Source: CAD feature listing. Evaluate the final solid. Frame: model axes, mm. A direction names the side the tool comes from. Give positions to 0.01 mm unless a question says otherwise; leave off trailing zeros. Write each loop counter-clockwise with the first axis right and the second up, starting at its lowest first coordinate (ties: lowest second). Pieces come first, ordered by that corner, then holes. Notation, with made-up numbers: (81, 23.25) - (111, 23.25) arc R12 ccw to (111, 35.25) - close; hole circle Ø3 at (66.5, 23). An arc over 180 degrees is marked (long way). One line per question, with ' | ' between items. Start each with the question number.
(1) Section C-C, the plane x = 50. Return loops of the section in (y, z).
(2) Access query for faces 4 (the flat face through (40.23, 0.99, -23.57)), 5 (the flat face through (41, 0, -24)). Directions: +Z, -Z, +X, -X, +Y, -Y. A direction counts if a zero-diameter tool reaches every point of the face in a straight line with its end or side. Return the directions, or none.
(3) Draft query along X for faces 1 (the flat face through (19.09, 0.99, -23.06)), 2 (the flat face through (44.5, 0.99, -26.18)), 3 (the flat face through (30, 1, 0)). Return one class per face: +X half, -X half, draft (parallel to the pull), parting line (faces both ways), or undercut.
(4) Ray query, line 1 (X direction, y = 0.9, z = -15.5); line 2 (X direction, y = 0.9, z = -25); line 3 (Z direction, x = 25, y = 0.7). Return the intervals inside material, ascending. Write a range as [from, to].
(5) Pin query (flat end, axial travel): pin 1 (12 mm diameter, centred on x = 29.5, z = -20, fed in from -Y); pin 2 (1 mm diameter, centred on x = 18.5, y = 0.5, fed in from -Z); pin 3 (1 mm diameter, centred on x = 26.5, y = 1.5, fed in from -Z). Return the tip coordinate at first contact, or that it passes through.
(6) Section B-B, the plane y = 1.4. Return loops of the section in (x, z), plus the area to 3 significant figures.
(7) Section A-A, the plane z = -8. Return loops of the section in (x, y), plus the area to 3 significant figures.
```python
from build123d import *

# Parameters (mm, degrees)
BOSS_EXTRUDE1_DEPTH = 2


with BuildPart() as part:
    # Sketch1 → Boss-Extrude1 (new body)
    with BuildSketch(Plane(origin=(0, 0, 0), x_dir=(1, 0, 0), z_dir=(0, 1, 0))):
        Polygon((0, 0), (29.8074, 51.627931242), (59.6148, 0), align=None)
        Polygon((50.9474, 5.004125723), (8.6674, 5.004125723), (29.8074, 41.619679795), align=None, mode=Mode.SUBTRACT)
    extrude(amount=BOSS_EXTRUDE1_DEPTH)


solid = part.part
```
Check sheet entries:
1) outline: (0, -16.65) - (2, -16.65) - (2, -6.65) - (0, -6.65) - close; (0, -5) - (2, -5) - (2, 0) - (0, 0) - close
2) face 4: +Y, -Y | face 5: +Z, -Z, +X, -X, -Y
3) face 1: undercut | face 2: +X half | face 3: draft
4) line 1: [8.95, 14.73], [44.89, 50.67] | line 2: [14.43, 20.21], [39.4, 45.18] | line 3: [-43.3, -33.29], [-5, 0]
5) pin 1: through | pin 2: z = -32.91 | pin 3: z = -46.77
6) outline: (0, 0) - (29.81, -51.63) - (59.61, 0) - close; hole (8.67, -5) - (29.81, -41.62) - (50.95, -5) - close | area: 765 mm²
7) outline: (4.62, 0) - (10.4, 0) - (10.4, 2) - (4.62, 2) - close; (49.22, 0) - (55, 0) - (55, 2) - (49.22, 2) - close | area: 23.1 mm²
